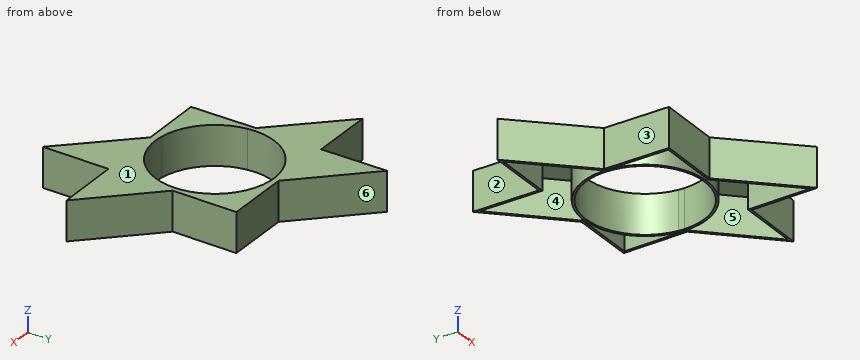
from build123d import *

# Parameters (mm, degrees)
F1_DEPTH = 45.72
F2_T     = -2.54


with BuildPart() as f1:
    # F0 (on Top) → F1 (new body)
    with BuildSketch(Plane.XY):
        Polygon((73.497205615, -75.4195482397), (148.5320329666, -74.2643550038), (74.735747165, 0.6356836955), align=None)
        with BuildLine():
            Line((73.497205615, -75.4195482397), (74.735747165, 0.6356836955))
            Line((74.735747165, 0.6356836955), (68.5921626755, 6.8711562673))
            ThreePointArc((68.5921626755, 6.8711562673), (68.8495817611, 3.4398634101), (68.9354594455, 0))
            ThreePointArc((68.9354594455, 0), (45.1804093562, -52.0656141744), (-9.7128356749, -68.247772067))
            Line((-9.7128356749, -68.247772067), (-1.652113798, -76.5765041298))
            Line((-1.652113798, -76.5765041298), (73.497205615, -75.4195482397))
        make_face()
        with BuildLine():
            Line((68.5921626755, 6.8711562673), (74.735747165, 0.6356836955))
            Line((74.735747165, 0.6356836955), (75.9635642171, 76.0323554277))
            Line((75.9635642171, 76.0323554277), (1.0778976806, 75.3952155197))
            Line((1.0778976806, 75.3952155197), (7.8886438881, 68.4826026562))
            ThreePointArc((7.8886438881, 68.4826026562), (49.1052036417, 48.3815723625), (68.5921626755, 6.8711562673))
        make_face()
        Polygon((72.235122323, -152.920410037), (73.497205615, -75.4195482397), (-1.652113798, -76.5765041298), align=None)
        with BuildLine():
            Line((-74.3026211858, -77.6949897408), (-1.652113798, -76.5765041298))
            Line((-1.652113798, -76.5765041298), (-9.7128356749, -68.247772067))
            ThreePointArc((-9.7128356749, -68.247772067), (-49.5352113263, -47.9412182554), (-68.5288572015, -7.4761821553))
            Line((-68.5288572015, -7.4761821553), (-74.3026211858, -1.5104468336))
            Line((-74.3026211858, -1.5104468336), (-74.3026211858, -77.6949897408))
        make_face()
        with BuildLine():
            ThreePointArc((-68.5288572015, -7.4761821553), (-48.5977686235, 48.891251301), (7.8886438881, 68.4826026562))
            Line((7.8886438881, 68.4826026562), (1.0778976806, 75.3952155197))
            Line((1.0778976806, 75.3952155197), (-74.3026211858, 74.7538653245))
            Line((-74.3026211858, 74.7538653245), (-74.3026211858, -1.5104468336))
            Line((-74.3026211858, -1.5104468336), (-68.5288572015, -7.4761821553))
        make_face()
        Polygon((-74.3026211858, 74.7538653245), (1.0778976806, 75.3952155197), (-74.3026211858, 151.9031822681), align=None)
        Polygon((-74.3026211858, -1.5104468336), (-74.3026211858, 74.7538653245), (-147.5100070238, 74.1310045123), align=None)
    extrude(amount=F1_DEPTH)

    # F2
    f2_openings = [f1.faces().sort_by_distance(p)[0] for p in [
        (108.607021, -39.796599, 0),
    ]]
    offset(amount=F2_T, openings=f2_openings, kind=Kind.INTERSECTION)


solid = f1.part
Work out the finished part from the listing and answer in its coordinate system (mm). Face numbers are marked on the shaded views. A direction names the side the tool comes from. Give positions to 0.01 mm unless a question says otherwise; leave off trailing zeros. Loops run counter-clockwise (first coordinate to the right, second up) from the corner with the lowest first, then second, coordinate; pieces in that order, holes last. Notation, with made-up numbers: M 6.25,-36.75 L 46.25,-36.75 A18 cw 46.25,-11.75 Z; hole C 55.5,-0.75 d11. An arc over 180 degrees is marked long. Use CSV: the item, a comma, the result in double quotes.
1) Consider L1, parallel to Y at x = 59, z = 36.5; L2, parallel to X at y = -51, z = 11; L3, parallel to Y at x = 5, z = 34.5. Determine where each line is inside the solid, lowest interval first.
Answer:
L1,"-139.25 to -135.59, -40.35 to -35.65, 35.65 to 40.35, 73.35 to 75.89"
L2,"-74.3 to -71.76, -50.08 to -46.38, 46.38 to 50.08, 122.04 to 125.61"
L3,"-83.45 to -79.8, -71.3 to -68.75, 68.75 to 71.3, 72.89 to 75.43"
2) Find section A-A on z = 6. Write down the section's boundary in (x, y), plus the area to 3 significant figures.
Answer:
outline,"M -147.51,74.13 L -74.3,-1.51 L -74.3,-77.69 L -1.65,-76.58 L 72.24,-152.92 L 73.5,-75.42 L 148.53,-74.26 L 74.74,0.64 L 75.96,76.03 L 1.08,75.4 L -74.3,151.9 L -74.3,74.75 Z; C 0,0 d142.95; hole M -141.57,71.64 L -71.76,-0.48 L -71.76,-75.12 L -0.59,-74.02 L 69.8,-146.75 L 71,-72.92 L 142.55,-71.82 L 72.18,-0.39 L 73.38,73.47 L 0.02,72.85 L -71.76,145.71 L -71.76,72.24 Z; hole C 0,0 d137.87"
area,"3,680 mm^2"
3) Find section C-C on y = -48.5. Write down the section's boundary in (x, z).
Answer:
outline,"M -74.3,0 L -71.76,0 L -71.76,43.18 L -52.5,43.18 L -52.5,0 L -48.99,0 L -48.99,45.72 L -74.3,45.72 Z; M 48.99,0 L 52.5,0 L 52.5,43.18 L 119.58,43.18 L 119.58,0 L 123.15,0 L 123.15,45.72 L 48.99,45.72 Z"
4) Given P1, Ø6, axis at x = 46, z = 5.5, coming from the -Y side; P2, Ø4, axis at x = 75.5, y = -50.5, coming from the -Z side; P3, Ø2, axis at y = 40, z = 36, coming from the -X side, each flat-ended and moving along its own axis, determine where each tip first touches the part or whether it passes through.
Answer:
P1,"y = -128.91"
P2,"z = 43.18"
P3,"x = -115.45"
5) Which of the six approach directions +Z, -Z, +X, -X, +Y, -Y give full straight-line access (tool end or side, diameter ignored) to the marked faces 1 and 2?
Answer:
face 1,"+Z, +X, -X, +Y, -Y"
face 2,"+Z, -Z, -X, +Y"
6) Determine the mould class of the marked faces 3, 4, 5 and 6 for opening direction Y: released by +Y, released by -Y, zero draft, split by the parting line, or undercut.
Answer:
face 3,"zero draft"
face 4,"undercut"
face 5,"undercut"
face 6,"released by +Y"
7) Find section D-D on x = 111.5. Write down the section's boundary in (y, z), plus the area to 3 significant figures.
Answer:
outline,"M -74.83,0 L -72.29,0 L -72.29,43.18 L -40.3,43.18 L -40.3,0 L -36.68,0 L -36.68,45.72 L -74.83,45.72 Z"
area,"363 mm^2"
8) Find section B-B on x = -38. Write down the section's boundary in (y, z).
Answer:
outline,"M -77.14,0 L -74.6,0 L -74.6,43.18 L -60.54,43.18 L -60.54,0 L -57.52,0 L -57.52,45.72 L -77.14,45.72 Z; M 57.52,0 L 60.54,0 L 60.54,43.18 L 111.44,43.18 L 111.44,0 L 115.06,0 L 115.06,45.72 L 57.52,45.72 Z"
